Source: CAD feature listing. Evaluate the final solid. Frame: model axes, mm. Round coordinates to 2 decimals unless told otherwise and drop trailing zeros. Order: outer loops, then holes, each group sorted by start corner. A loop starts at its lowest first (then second) coordinate and runs counter-clockwise, first axis right, second up. Notation, with made-up numbers: M -34,-38 L -19,-38 A16 ccw -19,-29 Z; hole C 56.5,-38.5 d5. An arc over 180 degrees is marked long. Answer in a Markdown table with one row per item. Add a question column.
```python
from build123d import *

# Parameters (mm, degrees)
RESSALTO_EXTRUS_O1_DEPTH = 2
CORTE_EXTRUS_O1_DEPTH    = 116.451288429


with BuildPart() as part:
    # Esboço1 → Ressalto-extrusão1 (new body)
    with BuildSketch(Plane(origin=(0, 0, 0), x_dir=(0, 0, -1), z_dir=(1, 0, 0))):
        with BuildLine():
            Line((0, 24.303568951), (0, 0.696431049))
            ThreePointArc((0, 0.696431049), (-0.203979932, 0.203979932), (-0.696431049, 0))
            Line((-0.696431049, 0), (-35.339881939, 0))
            ThreePointArc((-35.339881939, 0), (-35.806022669, 0.179005667), (-36.032536425, 0.624001989))
            ThreePointArc((-36.032536425, 0.624001989), (-37.984032615, 4.457802818), (-42, 6))
            Line((-42, 6), (-96, 6))
            Line((-96, 6), (-96.59021866, 9.347296355))
            ThreePointArc((-96.59021866, 9.347296355), (-98.907130521, 10.969615506), (-100.529449672, 8.652703645))
            Line((-100.529449672, 8.652703645), (-100.061706448, 6))
            Line((-100.061706448, 6), (-107, 6))
            ThreePointArc((-107, 6), (-109.918324731, 8.304744102), (-108.352654988, 11.677746157))
            Line((-108.352654988, 11.677746157), (-80.148093958, 25.925190806))
            ThreePointArc((-80.148093958, 25.925190806), (-79.995482912, 25.981039602), (-79.834083648, 26))
            Line((-79.834083648, 26), (-62, 26))
            ThreePointArc((-62, 26), (-60, 28), (-62, 30))
            Line((-62, 30), (-73.303568951, 30))
            ThreePointArc((-73.303568951, 30), (-73.796020068, 30.203979932), (-74, 30.696431049))
            Line((-74, 30.696431049), (-74, 34.303568951))
            ThreePointArc((-74, 34.303568951), (-73.796020068, 34.796020068), (-73.303568951, 35))
            Line((-73.303568951, 35), (-55.168160729, 35))
            ThreePointArc((-55.168160729, 35), (-55.004697711, 34.980544614), (-54.850367647, 34.92326546))
            Line((-54.850367647, 34.92326546), (-16, 15))
            ThreePointArc((-16, 15), (-13.465644125, 14.602459282), (-11.191291491, 15.789185206))
            ThreePointArc((-11.191291491, 15.789185206), (-10.963040008, 15.945135177), (-10.692099084, 16))
            Line((-10.692099084, 16), (-6, 16))
            ThreePointArc((-6, 16), (-4, 18), (-6, 20))
            Line((-6, 20), (-9.303568951, 20))
            ThreePointArc((-9.303568951, 20), (-9.796020068, 20.203979932), (-10, 20.696431049))
            Line((-10, 20.696431049), (-10, 24.303568951))
            ThreePointArc((-10, 24.303568951), (-9.796020068, 24.796020068), (-9.303568951, 25))
            Line((-9.303568951, 25), (-0.696431049, 25))
            ThreePointArc((-0.696431049, 25), (-0.203979932, 24.796020068), (0, 24.303568951))
        make_face()
        with BuildLine():
            Line((-92.308809913, 11), (-58.486017578, 11))
            ThreePointArc((-58.486017578, 11), (-57.155549564, 11.807284429), (-57.257169698, 13.360193517))
            Line((-57.257169698, 13.360193517), (-62.157169698, 20.360193517))
            ThreePointArc((-62.157169698, 20.360193517), (-62.693302007, 20.830468014), (-63.386017578, 21))
            Line((-63.386017578, 21), (-78.451452887, 21))
            ThreePointArc((-78.451452887, 21), (-78.799080836, 20.959162366), (-79.127780381, 20.838873079))
            Line((-79.127780381, 20.838873079), (-92.985137407, 13.838873079))
            ThreePointArc((-92.985137407, 13.838873079), (-93.767972278, 12.152372051), (-92.308809913, 11))
        make_face(mode=Mode.SUBTRACT)
    extrude(amount=RESSALTO_EXTRUS_O1_DEPTH)

    # Esboço2 → Corte-extrusão1 (cut, through all)
    with BuildSketch(Plane(origin=(2, 0, 0), x_dir=(0, 0, -1), z_dir=(1, 0, 0))):
        with BuildLine():
            Line((-40, 20.414213562), (-34, 14.414213562))
            ThreePointArc((-34, 14.414213562), (-34, 11.585786438), (-36.828427125, 11.585786438))
            Line((-36.828427125, 11.585786438), (-42.828427125, 17.585786438))
            ThreePointArc((-42.828427125, 17.585786438), (-42.828427125, 20.414213562), (-40, 20.414213562))
        make_face()
    extrude(amount=-CORTE_EXTRUS_O1_DEPTH, mode=Mode.SUBTRACT)


solid = part.part
```
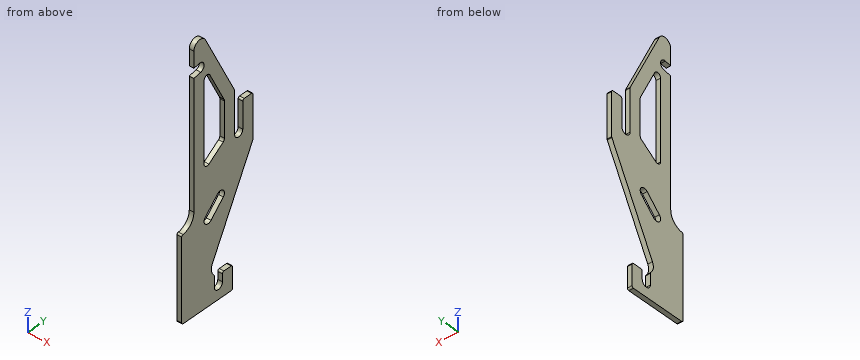
(1) Cut plane C-C (x = 0.3). Count the separate pieces of the cut face and the enclosed holes in it, and give its area (3 significant figures).
(2) Pin query (flat end, axial travel): pin 1 (8 mm diameter, centred on y = 27, z = 90, fed in from +X); pin 2 (1 mm diameter, centred on x = 1.5, z = 74, fed in from +Y); pin 3 (1 mm diameter, centred on x = 1, y = 25.5, fed in from +Z); pin 4 (1 mm diameter, centred on x = 1, z = 68, fed in from -Y). Return the tip coordinate at first contact, or that it passes through.
(3) Cut plane D-D (y = 28). Return loops of the section in (x, z).
(4) Line query: line 1 (Y direction, x = 0.6, z = 8); line 2 (Y direction, x = 1.3, z = 77); line 3 (Z direction, x = 1, y = 14.5). Output: solid intervals per line, ascending. Write a range as from..to.
(5) Cut plane B-B (y = 19). Return loops of the section in (x, z), and give its area (3 significant figures).
(6) Cut plane A-A (z = 86.5). Return loops of the section in (x, y), and give its area (3 significant figures).
Answer list:
| question | item | result |
|---|---|---|
| 1 | separate pieces | 1 |
| 1 | enclosed holes | 2 |
| 1 | area | 1,820 mm² |
| 2 | pin 1 | through |
| 2 | pin 2 | y = 34.97 |
| 2 | pin 3 | z = 81.98 |
| 2 | pin 4 | y = 6 |
| 3 | outline | M 0,41.35 L 2,41.35 L 2,60 L 0,60 Z |
| 4 | line 1 | 0..16, 20..25 |
| 4 | line 2 | 6..11, 21..26 |
| 4 | line 3 | 0..34.09, 39.74..58.06, 91.68..102.77 |
| 5 | outline | M 0,0 L 2,0 L 2,4.27 L 0,4.27 Z; M 0,23.8 L 2,23.8 L 2,38.59 L 0,38.59 Z; M 0,43.41 L 2,43.41 L 2,61.21 L 0,61.21 Z; M 0,82.77 L 2,82.77 L 2,93.86 L 0,93.86 Z |
| 5 | area | 95.9 mm² |
| 6 | outline | M 0,6 L 2,6 L 2,11 L 0,11 Z; M 0,17.11 L 2,17.11 L 2,22.72 L 0,22.72 Z |
| 6 | area | 21.2 mm² |
